Drawing for the job (mm, zero at the part's lowest x, y, z). A direction names the side the tool comes from. Round coordinates to 2 decimals unless told otherwise and drop trailing zeros. Order: outer loops, then holes, each group sorted by start corner. A loop starts at its lowest first (then second) coordinate and runs counter-clockwise, first axis right, second up. Notation, with made-up numbers: (-36.5, 89.5) - (-13.5, 89.5) arc R22 ccw to (-13.5, 117.5) - close; hole circle Ø9 at (81, -22). An arc over 180 degrees is marked (long way). Put each result on its own line as item: value. Start each with the question number.
Item 1: Probe probe 1 along Y at (x, z) = (52, 10); probe 2 along X at (y, z) = (11.75, 2.5); probe 3 along X at (y, z) = (6.25, 2.5). List the from-to ranges inside material, lowest first.
Item 2: Saw through at C-C on z = 11. List the corners of the cut face in (x, y), plus the area to 3 significant figures.
Item 3: Saw through at D-D on y = 18.5. List the corners of the cut face in (x, z).
Item 4: Mould opens along Z. For the marked faces 5, 6 and 7 say: pulls with the +Z half, pulls with the -Z half, needs draft (parallel to the pull), parting line crosses it, or undercut.
Item 5: Which spindle directions (+Z, -Z, +X, -X, +Y, -Y) get a long thin tool onto all of the face, cutting with end or side? Do the marked faces 1, 2, 3 and 4. Say none if no direction does.
Item 6: Saw through at A-A on y = 11.25. List the corners of the cut face in (x, z).
Item 7: Pin check, flat tips, straight feed: pin 1 Ø1.5 at (y, z) = (8, 17) entering from +X; pin 2 Ø16 at (y, z) = (21, 15) entering from -X; pin 3 Ø7.5 at (x, y) = (37, 12.5) entering from +Z. Stop position of each tip, or through.
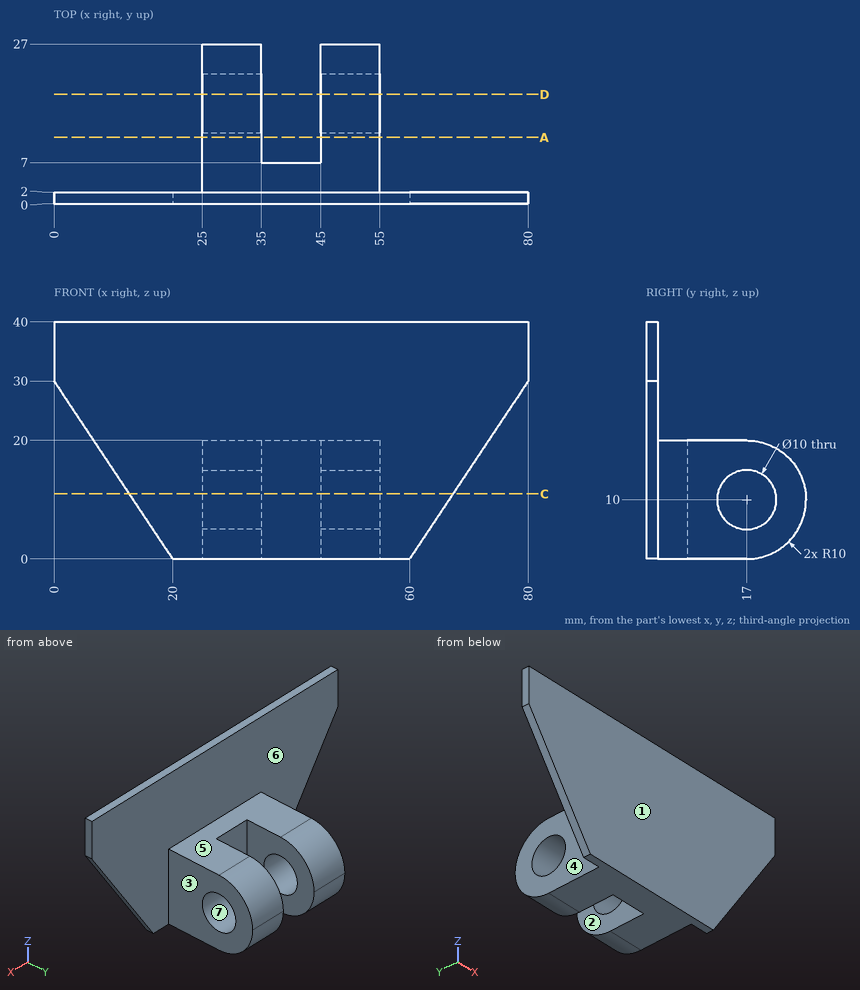
Results found:
1. probe 1: y = 0 to 12, 22 to 27
1. probe 2: x = 25 to 35, 45 to 55
1. probe 3: x = 25 to 55
2. outline: (12.67, 0) - (67.33, 0) - (67.33, 2) - (55, 2) - (55, 12.1) - (45, 12.1) - (45, 7) - (35, 7) - (35, 12.1) - (25, 12.1) - (25, 2) - (12.67, 2) - close; (25, 21.9) - (35, 21.9) - (35, 26.95) - (25, 26.95) - close; (45, 21.9) - (55, 21.9) - (55, 26.95) - (45, 26.95) - close
2. area: 462 mm²
3. outline: (25, 0.11) - (35, 0.11) - (35, 5.23) - (25, 5.23) - close; (25, 14.77) - (35, 14.77) - (35, 19.89) - (25, 19.89) - close; (45, 0.11) - (55, 0.11) - (55, 5.23) - (45, 5.23) - close; (45, 14.77) - (55, 14.77) - (55, 19.89) - (45, 19.89) - close
4. face 5: pulls with the +Z half
4. face 6: needs draft
4. face 7: undercut
5. face 1: +Z, -Z, +X, -X, -Y
5. face 2: +Z, -Z, +Y
5. face 3: +Z, -Z, +X, +Y
5. face 4: +Z, -Z, -X, +Y
6. outline: (25, 0) - (35, 0) - (35, 20) - (25, 20) - close; (45, 0) - (55, 0) - (55, 20) - (45, 20) - close
7. pin 1: stops at x = 55
7. pin 2: stops at x = 25
7. pin 3: stops at z = 20
